from build123d import *

# Parameters (mm, degrees)
HIERRO_ANGULAR_2_X_2_X_0_125_1_DEPTH = 50.8
CROQUIS3_R                           = 4.5
CORTAR_EXTRUIR1_DEPTH                = 10


with BuildPart() as part:
    # Sketch1 → Hierro angular 2 X 2 X 0.125(1) (new body)
    with BuildSketch(Plane(origin=(0, 0, 0), x_dir=(-1, 0, 0), z_dir=(0, 1, 0))):
        with BuildLine():
            Line((0, 0), (0, 50.8))
            Line((0, 50.8), (0.00508, 50.8))
            ThreePointArc((0.00508, 50.8), (2.246551928, 49.871551928), (3.175, 47.63008))
            Line((3.175, 47.63008), (3.175, 7.9375))
            ThreePointArc((3.175, 7.9375), (4.569903955, 4.569903955), (7.9375, 3.175))
            Line((7.9375, 3.175), (47.63008, 3.175))
            ThreePointArc((47.63008, 3.175), (49.871551928, 2.246551928), (50.8, 0.00508))
            Line((50.8, 0.00508), (50.8, 0))
            Line((50.8, 0), (0, 0))
        make_face()
    extrude(amount=HIERRO_ANGULAR_2_X_2_X_0_125_1_DEPTH)

    # Croquis3 → Cortar-Extruir1 (cut)
    with BuildSketch(Plane.XY.offset(3.175)):
        with Locations((-32.63008, 25.4)):
            Circle(CROQUIS3_R)
    extrude(amount=-CORTAR_EXTRUIR1_DEPTH, mode=Mode.SUBTRACT)


solid = part.part
Design review of the part built by this model. Coordinates are the model's own, in mm. A direction names the side the tool comes from. Give positions to 0.01 mm unless a question says otherwise; leave off trailing zeros. Order: outer loops, then holes, each group sorted by start corner. A loop starts at its lowest first (then second) coordinate and runs counter-clockwise, first axis right, second up.
1. Tool access review of faces 1 (the flat face through (-26, 25, 0)), 2 (the flat face through (-27.5, 25, 3.175)): name each direction out of +Z, -Z, +X, -X, +Y, -Y from which nothing blocks a thin tool from reaching the whole face with its end or side.
Solution:
face 1: -Z, +X, -X, +Y, -Y
face 2: +Z, -X, +Y, -Y
2. Mouldability with a two-part tool opening along Y and no side actions: class faces 3 (the cylindrical face through (-36.2, 22.66, 1.61)), 4 (the flat face through (-14, 0, 3)), 5 (the cylindrical face through (-2.22, 25.04, 49.9)) as +Y half, -Y half, draft (parallel to the pull), parting line (faces both ways), or undercut.
Solution:
face 3: undercut
face 4: -Y half
face 5: draft
3. To check wall thickness, follow L1, parallel to Z at x = -17, y = 36 (3 decimals); L2, parallel to X at y = 4, z = 25 (3 decimals); L3, parallel to X at y = 25, z = 1. State the ranges of each line that lie inside material, in increasing order.
Solution:
L1: z = 0 to 3.175
L2: x = -3.175 to 0
L3: x = -50.64 to -37.11, -28.15 to 0
4. Add section D-D, the plane z = 25.5. State the section outline as (x, y) points (3 decimals), then the cut area to 3 significant figures.
Solution:
outline: (-3.175, 0) - (0, 0) - (0, 50.8) - (-3.175, 50.8) - close
area: 161 mm2
5. For pin 1 Ø8 at (y, z) = (29.5, 27) entering from -X (3 decimals); pin 2 Ø6 at (x, y) = (-21.5, 44.5) entering from +Z (3 decimals); pin 3 Ø5.5 at (x, y) = (-32.63, 25.4) entering from -Z, all flat-tipped, find the tip position at first contact; note any pin that passes through.
Solution:
pin 1: stops at x = -3.175
pin 2: stops at z = 3.175
pin 3: passes through
6. Add section C-C, the plane x = -20. State the section outline as (y, z) points (3 decimals), then the cut area to 3 significant figures.
Solution:
outline: (0, 0) - (50.8, 0) - (50.8, 3.175) - (0, 3.175) - close
area: 161 mm2
